```python
from build123d import *

# Parameters (mm, degrees)
BOSS_EXTRUDE1_DEPTH     = 45
SKETCH3_OUTSIDE_W       = 76.716
SKETCH3_OUTSIDE_H       = 76.716
CUT_EXTRUDE1_DEPTH      = 40
SKETCH4_R               = 2.5
CUT_EXTRUDE3_DEPTH      = 46
CUT_EXTRUDE3_DEPTH_BACK = 1
SKETCH5_R               = 19
BOSS_EXTRUDE2_DEPTH     = 1.5
SKETCH6_R               = 3
BOSS_EXTRUDE3_DEPTH     = 18.5


with BuildPart() as part:
    # Sketch2 → Boss-Extrude1 (new body)
    with BuildSketch(Plane(origin=(0, 0, 0), x_dir=(1, 0, 0), z_dir=(0, 1, 0))):
        with BuildLine():
            Line((-28.2, -23.2), (-28.2, 23.2))
            ThreePointArc((-28.2, 23.2), (-26.735533906, 26.735533906), (-23.2, 28.2))
            Line((-23.2, 28.2), (23.2, 28.2))
            ThreePointArc((23.2, 28.2), (26.735533906, 26.735533906), (28.2, 23.2))
            Line((28.2, 23.2), (28.2, -23.2))
            ThreePointArc((28.2, -23.2), (26.735533906, -26.735533906), (23.2, -28.2))
            Line((23.2, -28.2), (-23.2, -28.2))
            ThreePointArc((-23.2, -28.2), (-26.735533906, -26.735533906), (-28.2, -23.2))
        make_face()
    extrude(amount=BOSS_EXTRUDE1_DEPTH)

    # Sketch3 outside → Cut-Extrude1 (cut)
    with BuildSketch(Plane.XZ):
        Rectangle(SKETCH3_OUTSIDE_W, SKETCH3_OUTSIDE_H)
        with BuildLine():
            Line((-28.2, 17.57), (-23.57, 17.57))
            ThreePointArc((-23.57, 17.57), (-19.327359313, 19.327359313), (-17.57, 23.57))
            Line((-17.57, 23.57), (-17.57, 28.2))
            Line((-17.57, 28.2), (17.57, 28.2))
            Line((17.57, 28.2), (17.57, 23.57))
            ThreePointArc((17.57, 23.57), (19.327359313, 19.327359313), (23.57, 17.57))
            Line((23.57, 17.57), (28.2, 17.57))
            Line((28.2, 17.57), (28.2, -17.57))
            Line((28.2, -17.57), (23.57, -17.57))
            ThreePointArc((23.57, -17.57), (19.327359313, -19.327359313), (17.57, -23.57))
            Line((17.57, -23.57), (17.57, -28.2))
            Line((17.57, -28.2), (-17.57, -28.2))
            Line((-17.57, -28.2), (-17.57, -23.57))
            ThreePointArc((-17.57, -23.57), (-19.327359313, -19.327359313), (-23.57, -17.57))
            Line((-23.57, -17.57), (-28.2, -17.57))
            Line((-28.2, -17.57), (-28.2, 17.57))
        make_face(mode=Mode.SUBTRACT)
    extrude(amount=-CUT_EXTRUDE1_DEPTH, mode=Mode.SUBTRACT)

    # Sketch4 → Cut-Extrude3 (cut, two sides)
    with BuildSketch(Plane(origin=(0, 0, 0), x_dir=(1, 0, 0), z_dir=(0, 1, 0))) as cut_extrude3_sk:
        with Locations((23.57, -23.57)):
            Circle(SKETCH4_R)
        with Locations((-23.57, -23.57)):
            Circle(SKETCH4_R)
        with Locations((23.57, 23.57)):
            Circle(SKETCH4_R)
        with Locations((-23.57, 23.57)):
            Circle(SKETCH4_R)
    extrude(amount=CUT_EXTRUDE3_DEPTH, mode=Mode.SUBTRACT)
    extrude(cut_extrude3_sk.sketch, amount=-CUT_EXTRUDE3_DEPTH_BACK, mode=Mode.SUBTRACT)

    # Sketch5 → Boss-Extrude2 (add)
    with BuildSketch(Plane(origin=(0, 45, 0), x_dir=(1, 0, 0), z_dir=(0, 1, 0))):
        Circle(SKETCH5_R)
    extrude(amount=BOSS_EXTRUDE2_DEPTH)

    # Sketch6 → Boss-Extrude3 (add)
    with BuildSketch(Plane(origin=(0, 46.5, 0), x_dir=(1, 0, 0), z_dir=(0, 1, 0))):
        Circle(SKETCH6_R)
    extrude(amount=BOSS_EXTRUDE3_DEPTH)


solid = part.part
```
Can you work these out from the model? Positions are in its coordinate system, mm. A direction names the side the tool comes from. Coordinates: 2 decimals unless noted, no trailing zeros. Loops run counter-clockwise (first coordinate to the right, second up) from the corner with the lowest first, then second, coordinate; pieces in that order, holes last. Notation, with made-up numbers: (-36.5, 7) -> (22.5, 7) arc R15 ccw to (22.5, 22) -> close; hole circle Ø8 at (59, -36.5). An arc over 180 degrees is marked (long way). Answer as a JSON object with one key per item and string values.
1) If I drill on line 1 (Z direction, x = -23.57, y = 43.45); line 2 (X direction, y = 41, z = 23), over which ranges is the centre line in solid material (lowest first)?
Results:
{"line 1": "z = -28.19 to -26.07, -21.07 to 21.07, 26.07 to 28.19", "line 2": "x = -28.2 to -26, -21.14 to 21.14, 26 to 28.2"}
2) For P1, Ø17, axis at x = -12, z = 12.5, coming from the +Y side; P2, Ø3.5, axis at x = 26.5, y = 20, coming from the -Z side; P3, Ø3.5, axis at y = 19, z = 26, coming from the -X side, each with a flat end and sliding along its axis, tell me the tip position at first contact or that it passes through.
Results:
{"P1": "stops at y = 46.5", "P2": "stops at z = -17.57", "P3": "stops at x = -17.57"}
3) Imagine slicing it at C-C (z = 0). Please give me the cut outline in (x, y).
Results:
{"outline": "(-28.2, 0) -> (28.2, 0) -> (28.2, 45) -> (19, 45) -> (19, 46.5) -> (3, 46.5) -> (3, 65) -> (-3, 65) -> (-3, 46.5) -> (-19, 46.5) -> (-19, 45) -> (-28.2, 45) -> close"}
4) Imagine slicing it at B-B (x = 0). Please give me the cut outline in (y, z), then the cut area to 3 significant figures.
Results:
{"outline": "(0, -28.2) -> (45, -28.2) -> (45, -19) -> (46.5, -19) -> (46.5, -3) -> (65, -3) -> (65, 3) -> (46.5, 3) -> (46.5, 19) -> (45, 19) -> (45, 28.2) -> (0, 28.2) -> close", "area": "2,710 mm^2"}
5) Imagine slicing it at A-A (y = 41). Please give me the cut outline in (x, z).
Results:
{"outline": "(-28.2, -23.2) arc R5 ccw to (-23.2, -28.2) -> (23.2, -28.2) arc R5 ccw to (28.2, -23.2) -> (28.2, 23.2) arc R5 ccw to (23.2, 28.2) -> (-23.2, 28.2) arc R5 ccw to (-28.2, 23.2) -> close; hole circle Ø5 at (-23.57, -23.57); hole circle Ø5 at (-23.57, 23.57); hole circle Ø5 at (23.57, -23.57); hole circle Ø5 at (23.57, 23.57)"}
6) Thinking about a two-plate mould opening in X: for faces 1 (the face through (-23, 40, -20)), 2 (the face through (-17.57, 20, -26)), 3 (the face through (21.73, 42.46, -25.26)), which applies, pulls with the +X half, pulls with the -X half, needs draft (parallel to the pull), parting line crosses it, or undercut?
Results:
{"face 1": "needs draft", "face 2": "pulls with the -X half", "face 3": "undercut"}
7) Imagine slicing it at D-D (y = 33). Please give me the cut outline in (x, z), then the cut area to 3 significant figures.
Results:
{"outline": "(-28.2, -17.57) -> (-23.57, -17.57) arc R6 cw to (-17.57, -23.57) -> (-17.57, -28.2) -> (17.57, -28.2) -> (17.57, -23.57) arc R6 cw to (23.57, -17.57) -> (28.2, -17.57) -> (28.2, 17.57) -> (23.57, 17.57) arc R6 cw to (17.57, 23.57) -> (17.57, 28.2) -> (-17.57, 28.2) -> (-17.57, 23.57) arc R6 cw to (-23.57, 17.57) -> (-28.2, 17.57) -> close", "area": "2,760 mm^2"}
8) For faces 4 (the face through (8.767, 45.74, 16.856)), 5 (the face through (21.6, 40, -21.6)), 6 (the face through (20, 40, 23)), 7 (the face through (-26, 20, 17.57)), which set-ups out of +Z, -Z, +X, -X, +Y, -Y let a thin tool reach every point of the face, with its end or its side?
Results:
{"face 4": "+Y", "face 5": "-Z, +X, -Y", "face 6": "+Z, +X, -Y", "face 7": "+Z, -X, -Y"}
